from build123d import *

# Parameters (mm, degrees)
F0_W     = 27.94
F0_H     = 38.1
F1_DEPTH = 25.4
F3_T     = -2.54
F2_W     = 4.064
F2_H     = 5.08
F4_DEPTH = 25.4


with BuildPart() as f1:
    # F0 (on Top) → F1 (new body)
    with BuildSketch(Plane.XY):
        Rectangle(F0_W, F0_H)
    extrude(amount=F1_DEPTH)

    # F3
    f3_openings = [f1.faces().sort_by_distance(p)[0] for p in [
        (0, -19.05, 12.7),
        (0, 0, 0),
        (0, 19.05, 12.7),
    ]]
    offset(amount=F3_T, openings=f3_openings)

    # F2 (on face) → F4 (cut)
    with BuildSketch(Plane.XY.offset(25.4)):
        with Locations((0, 11.43)):
            Rectangle(F2_W, F2_H)
        with Locations((-6.35, -11.43)):
            Rectangle(F2_W, F2_H)
        with Locations((6.35, -11.43)):
            Rectangle(F2_W, F2_H)
    extrude(amount=-F4_DEPTH, mode=Mode.SUBTRACT)


solid = f1.part
Geometry check sheet. Reference: the model listing, model coordinates, mm. A direction names the side the tool comes from. Coordinates: 2 decimals unless noted, no trailing zeros. Order: outer loops, then holes, each group sorted by start corner. A loop starts at its lowest first (then second) coordinate and runs counter-clockwise, first axis right, second up. Notation, with made-up numbers: (60, 17.5) - (66, 17.5) arc R20 ccw to (66, 42.5) - close; hole circle Ø8 at (59.25, 78.25). An arc over 180 degrees is marked (long way). Answer in a Markdown table with one row per item. Add a question column.
1) Material ranges on line 1 along X through (y, z) = (-9.5, 5.25); line 2 along Z through (x, y) = (0, 3.5), recorded low to high. Write a range as [from, to].
2) Set-up check for faces 1 (the flat face through (13.97, 0, 13)), 2 (the flat face through (6, -8.89, 24)), 3 (the flat face through (0, 0, 22.86)): record each of +Z, -Z, +X, -X, +Y, -Y from which the full face is reachable in a straight line by a thin tool's end or side.
3) Cross-section at A-A, the plane x = 7.75. Record the cut outline in (y, z).
4) Cross-section at C-C, the plane y = -2.5. Record the cut outline in (x, z), then the cut area to 3 significant figures.
5) Cross-section at B-B, the plane z = 9.75. Record the cut outline in (x, y).
6) Cross-section at D-D, the plane x = 11. Record the cut outline in (y, z), then the cut area to 3 significant figures.
7) Release check for a two-part mould opening along Y. For faces 4 (the flat face through (0, 8.89, 24)), 5 (the flat face through (-11.43, 0, 11)) record: +Y half, -Y half, draft (parallel to the pull), parting line (faces both ways), or undercut.
8) Gauge pin test, flat ends, axial feed: P1, Ø10, axis at x = 10.5, z = 3, coming from the +Y side; P2, Ø2, axis at x = -0.5, y = 6.5, coming from the -Z side. Record the tip position at first contact, or that the pin passes through.
Check result:
| question | item | result |
|---|---|---|
| 1 | line 1 | x = [-13.97, -11.43], [11.43, 13.97] |
| 1 | line 2 | z = [22.86, 25.4] |
| 2 | face 1 | +Z, -Z, +X, +Y, -Y |
| 2 | face 2 | +Z, -Z |
| 2 | face 3 | -Z, +Y, -Y |
| 3 | outline | (-19.05, 22.86) - (-13.97, 22.86) - (-13.97, 25.4) - (-19.05, 25.4) - close; (-8.89, 22.86) - (19.05, 22.86) - (19.05, 25.4) - (-8.89, 25.4) - close |
| 4 | outline | (-13.97, 0) - (-11.43, 0) - (-11.43, 22.86) - (11.43, 22.86) - (11.43, 0) - (13.97, 0) - (13.97, 25.4) - (-13.97, 25.4) - close |
| 4 | area | 187 mm² |
| 5 | outline | (-13.97, -19.05) - (-11.43, -19.05) - (-11.43, 19.05) - (-13.97, 19.05) - close; (11.43, -19.05) - (13.97, -19.05) - (13.97, 19.05) - (11.43, 19.05) - close |
| 6 | outline | (-19.05, 22.86) - (19.05, 22.86) - (19.05, 25.4) - (-19.05, 25.4) - close |
| 6 | area | 96.8 mm² |
| 7 | face 4 | undercut |
| 7 | face 5 | draft |
| 8 | P1 | stops at y = 19.05 |
| 8 | P2 | stops at z = 22.86 |
